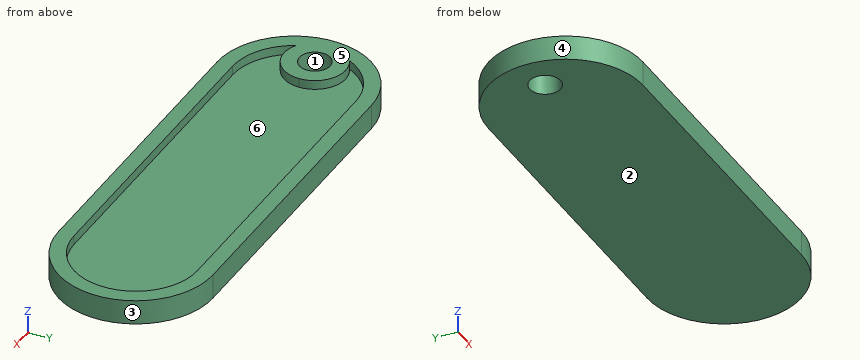
from build123d import *

# Parameters (mm, degrees)
F1_DEPTH = 4
F3_DEPTH = 1.5
F5_DEPTH = 1.5
F6_DEPTH = 1.5
F7_R     = 2.5
F8_DEPTH = 25


with BuildPart() as f1:
    # F0 (on Top) → F1 (new body)
    with BuildSketch(Plane.XY):
        with BuildLine():
            ThreePointArc((12.5, 25), (0, 12.5), (12.5, 0))
            Line((12.5, 0), (62.5, 0))
            ThreePointArc((62.5, 0), (75, 12.5), (62.5, 25))
            Line((62.5, 25), (12.5, 25))
        make_face()
    extrude(amount=F1_DEPTH)

    # F2 (on face) → F3 (cut)
    with BuildSketch(Plane.XY.offset(4)):
        with BuildLine():
            Line((62.5, 22.5), (12.5, 22.5))
            ThreePointArc((12.5, 22.5), (2.5, 12.5), (12.5, 2.5))
            Line((12.5, 2.5), (62.5, 2.5))
            ThreePointArc((62.5, 2.5), (72.5, 12.5), (62.5, 22.5))
        make_face()
    extrude(amount=-F3_DEPTH, mode=Mode.SUBTRACT)

    # F4 (on face) → F5 (join)
    with BuildSketch(Plane.XY.offset(2.5)):
        with BuildLine():
            ThreePointArc((3.4807692308, 8.1810329555), (2.5, 12.5), (3.4807692308, 16.8189670445))
            ThreePointArc((3.4807692308, 16.8189670445), (1, 12.5), (3.4807692308, 8.1810329555))
        make_face()
    extrude(amount=F5_DEPTH)

    # F4 (on face) → F6 (join)
    with BuildSketch(Plane.XY.offset(2.5)):
        with BuildLine():
            ThreePointArc((3.4807692308, 8.1810329555), (8.4903660528, 8.1643250902), (11, 12.5))
            ThreePointArc((11, 12.5), (8.4903660528, 16.8356749098), (3.4807692308, 16.8189670445))
            ThreePointArc((3.4807692308, 16.8189670445), (2.5, 12.5), (3.4807692308, 8.1810329555))
        make_face()
    extrude(amount=F6_DEPTH)

    # F7 (on face) → F8 (cut)
    with BuildSketch(Plane.XY.offset(4)):
        with Locations((6, 12.5)):
            Circle(F7_R)
    extrude(amount=-F8_DEPTH, mode=Mode.SUBTRACT)


solid = f1.part
The model under review builds one solid part; all positions refer to its coordinate system, in mm. Face numbers are marked on the shaded views. A direction names the side the tool comes from. Round coordinates to 2 decimals unless told otherwise and drop trailing zeros. Order: outer loops, then holes, each group sorted by start corner. A loop starts at its lowest first (then second) coordinate and runs counter-clockwise, first axis right, second up. Notation, with made-up numbers: (-12.75, -22) -> (-5.75, -22) arc R37 cw to (-5.75, 16) -> close; hole circle Ø9 at (72, 4.5). An arc over 180 degrees is marked (long way). Write item = value, one per line. Start each with the question number.
Item 1: Consider section B-B on x = 14.5. Write out the cut boundary in (y, z).
Item 2: Mouldability with a two-part tool opening along X and no side actions: class the marked faces 1, 2, 3 and 4 as released by +X, released by -X, zero draft, split by the parting line, or undercut.
Item 3: Consider section D-D on y = 19.5. Write out the cut boundary in (x, z), plus the area to 3 significant figures.
Item 4: Consider section A-A on x = 6. Write out the cut boundary in (y, z).
Item 5: For the marked faces 5 and 6, list the 3-axis set-ups (+Z, -Z, +X, -X, +Y, -Y) from which the entire face can be reached by the end or side of a thin tool; tool diameter is ignored.
Item 6: Consider section C-C on z = 1.45. Write out the cut boundary in (x, y), plus the area to 3 significant figures.
Item 7: For line 1 along Y through (x, z) = (10.5, 2.7); line 2 along Y through (x, z) = (6, 2.75); line 3 along Z through (x, y) = (63.5, 20.75), list the stretches that pass through material, from the lowest coordinate up.
Item 8: Clearance check with a flat-ended pin moving along its axis: pin 1 Ø3 at (x, y) = (52, 8.5) entering from +Z. State where the tip first meets the part, or that it passes through.
Conclusion:
q1.outline = (0, 0) -> (25, 0) -> (25, 4) -> (22.5, 4) -> (22.5, 2.5) -> (2.5, 2.5) -> (2.5, 4) -> (0, 4) -> close
q2.face_1 = undercut
q2.face_2 = zero draft
q2.face_3 = released by +X
q2.face_4 = released by -X
q3.outline = (2.14, 0) -> (72.86, 0) -> (72.86, 4) -> (69.64, 4) -> (69.64, 2.5) -> (5.36, 2.5) -> (5.36, 4) -> (2.14, 4) -> close
q3.area = 186 mm2
q4.outline = (1.82, 0) -> (10, 0) -> (10, 4) -> (7.5, 4) -> (7.5, 2.5) -> (4.9, 2.5) -> (4.9, 4) -> (1.82, 4) -> close; (15, 0) -> (23.18, 0) -> (23.18, 4) -> (20.1, 4) -> (20.1, 2.5) -> (17.5, 2.5) -> (17.5, 4) -> (15, 4) -> close
q5.face_5 = +Z, +X, -X, +Y, -Y
q5.face_6 = +Z
q6.outline = (12.5, 0) -> (62.5, 0) arc R12.5 ccw to (62.5, 25) -> (12.5, 25) arc R12.5 ccw to start; hole circle Ø5 at (6, 12.5)
q6.area = 1,720 mm2
q7.line_1 = 0.16 to 2.7, 10.32 to 14.68, 22.3 to 24.84
q7.line_2 = 1.82 to 4.9, 7.5 to 10, 15 to 17.5, 20.1 to 23.18
q7.line_3 = 0 to 2.5
q8.pin_1 = 2.5
